Can you work these out from the model? Positions are in its coordinate system, mm. Face numbers are marked on the shaded views. A direction names the side the tool comes from. Give positions to 0.01 mm unless a question says otherwise; leave off trailing zeros. Order: outer loops, then holes, each group sorted by start corner. A loop starts at its lowest first (then second) coordinate and runs counter-clockwise, first axis right, second up. Notation, with made-up numbers: M 67.25,56 L 101.25,56 A28 cw 101.25,74 Z; hole C 72.5,46 d4. An arc over 180 degrees is marked long. Write each question's results on one line, items separated by ' | '.
from build123d import *

# Parameters (mm, degrees)
BOSS_EXTRUDE1_DEPTH     = 25
CUT_EXTRUDE1_DEPTH      = 6
CUT_EXTRUDE1_DEPTH_BACK = 6
SKETCH2_R               = 2.65
SKETCH3_R               = 2.65
CUT_EXTRUDE2_DEPTH      = 91.385151574
CHAMFER1_SIZE           = 10
SKETCH4_R               = 5
CUT_EXTRUDE4_DEPTH      = 6
CHAMFER2_SIZE           = 10
SKETCH5_R               = 5
CUT_EXTRUDE5_DEPTH      = 6


with BuildPart() as part:
    # Sketch1 → Boss-Extrude1 (new body)
    with BuildSketch(Plane(origin=(0, 0, 0), x_dir=(0, 0, -1), z_dir=(1, 0, 0))):
        Polygon((0, 0), (0, 10), (-20, 10), (-20, 14), (0, 14), (0, 84.525), (20, 84.525), (20, 80.525), (4, 80.525), (4, 70), (20, 70), (20, 66), (4, 66), (4, 0), align=None)
    extrude(amount=BOSS_EXTRUDE1_DEPTH)

    # Sketch2 → Cut-Extrude1 (cut, two sides: drawn at the far end of the back side and taken through both)
    with BuildSketch(Plane(origin=(0, 14, 0), x_dir=(1, 0, 0), z_dir=(0, 1, 0)).offset(-CUT_EXTRUDE1_DEPTH_BACK)):
        with Locations(Location((12.5, -10, 0), (0, 0, 90))):
            Circle(SKETCH2_R)
    extrude(amount=CUT_EXTRUDE1_DEPTH + CUT_EXTRUDE1_DEPTH_BACK, mode=Mode.SUBTRACT)

    # Sketch3 → Cut-Extrude2 (cut, through all)
    with BuildSketch(Plane(origin=(0, 84.525, 0), x_dir=(1, 0, 0), z_dir=(0, 1, 0))):
        with Locations(Location((12.5, 14, 0), (0, 0, 270))):
            Circle(SKETCH3_R)
    extrude(amount=-CUT_EXTRUDE2_DEPTH, mode=Mode.SUBTRACT)

    # Chamfer1
    # the kernel refuses this chamfer: 10 mm, written as the material it adds along each edge
    with BuildSketch(Plane(origin=(0, 14, 0), x_dir=(0, -0.027495876610586317, 0.9996219169112968), z_dir=(1, 0, 0))) as chamfer1_piece_1_section:
        Polygon((CHAMFER1_SIZE * 0.999621916911, -CHAMFER1_SIZE * 0.0274958766106), (-CHAMFER1_SIZE * 0.0274958766106, -CHAMFER1_SIZE * 0.999621916911), (0, 0), align=None)
    chamfer1_piece_1 = extrude(amount=25, mode=Mode.PRIVATE)
    chamfer1_piece_1 = chamfer1_piece_1 - Plane(origin=(12.5, 17.333000487, 10), x_dir=(0, 0, -1), z_dir=(0, 1, 0)) * Cylinder(2.65, 90, mode=Mode.PRIVATE)
    add(chamfer1_piece_1)

    # Sketch4 → Cut-Extrude4 (cut)
    with BuildSketch(Plane(origin=(0, 14, 0), x_dir=(1, 0, 0), z_dir=(0, 1, 0))):
        with Locations((12.5, -10)):
            Circle(SKETCH4_R)
    extrude(amount=CUT_EXTRUDE4_DEPTH, mode=Mode.SUBTRACT)

    # Chamfer2
    # the kernel refuses this chamfer: 10 mm, written as the material it adds along each edge
    with BuildSketch(Plane(origin=(0, 66, -4), x_dir=(0, -0.9996219169112968, 0.027495876610586233), z_dir=(1, 0, 0))) as chamfer2_piece_1_section:
        Polygon((CHAMFER2_SIZE * 0.999621916911, CHAMFER2_SIZE * 0.0274958766106), (-CHAMFER2_SIZE * 0.0274958766106, CHAMFER2_SIZE * 0.999621916911), (0, 0), align=None)
    chamfer2_piece_1 = extrude(amount=25, mode=Mode.PRIVATE)
    chamfer2_piece_1 = chamfer2_piece_1 - Plane(origin=(12.5, 62.667000224, -14), x_dir=(0, 0, 1), z_dir=(0, 1, 0)) * Cylinder(2.65, 90, mode=Mode.PRIVATE)
    add(chamfer2_piece_1)

    # Sketch5 → Cut-Extrude5 (cut)
    with BuildSketch(Plane.XZ.offset(-66)):
        with Locations((12.5, -14)):
            Circle(SKETCH5_R)
    extrude(amount=CUT_EXTRUDE5_DEPTH, mode=Mode.SUBTRACT)


solid = part.part
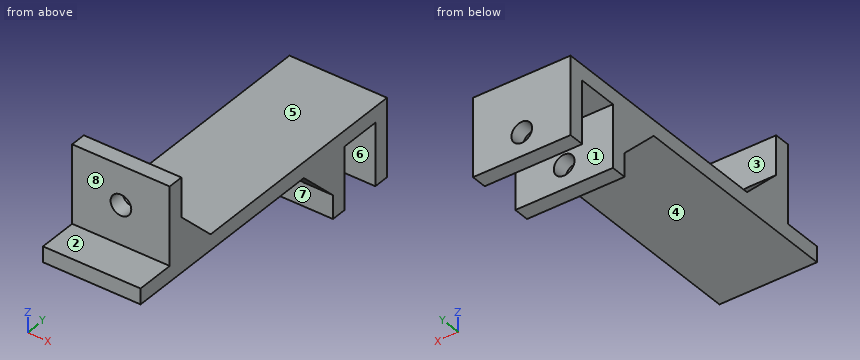
(1) We'd pull the mould along Y, two halves only. Please class the marked faces 1, 2 and 3: +Y half, -Y half, draft (parallel to the pull), parting line (faces both ways), or undercut.
Data:
face 1: undercut | face 2: draft | face 3: +Y half
(2) I need wall thicknesses on L1, parallel to X at y = 68.05, z = -14; L2, parallel to Z at x = 13.75, y = 9; L3, parallel to Y at x = 3.25, z = 5. Which ranges of each line are inside material? Lowest first, please. Write a range as from..to.
Data:
L1: x = 0..9.85, 15.15..25 | L2: z = -4..0 | L3: y = 10..19
(3) Imagine slicing it at B-B, the plane y = 12.5. Write out the boundary of the cut face in (x, z).
Data:
outline: M 0,-4 L 25,-4 L 25,20 L 0,20 Z; hole C 12.5,10 d5.3
(4) Imagine slicing it at A-A, the plane x = 12.5. Count the separate pieces of the cut face and the enclosed holes in it, plus the area to 4 significant figures.
Data:
separate pieces: 4 | enclosed holes: 0 | area: 557.5 mm2
(5) Will these pins go through, and if not, where does the flat tip stop? P1, Ø5, axis at x = 14.5, y = 7, coming from the +Z side; P2, Ø12, axis at x = 8.5, z = 13, coming from the -Y side; P3, Ø1.5, axis at x = 17, z = -15, coming from the -Y side.
Data:
P1: stops at z = 0 | P2: stops at y = 10 | P3: stops at y = 66
(6) Imagine slicing it at D-D, the plane x = 18.5. Write out the boundary of the cut face in (y, z) (3 decimals), plus the area to 3 significant figures.
Data:
outline: M 0,-4 L 56,-4 L 66,-14 L 66,-20 L 70,-20 L 70,-4 L 80.525,-4 L 80.525,-20 L 84.525,-20 L 84.525,0 L 24,0 L 14,10 L 14,20 L 10,20 L 10,0 L 0,0 Z | area: 646 mm2
(7) Imagine slicing it at C-C, the plane z = 9. Write out the boundary of the cut face in (x, y).
Data:
outline: M 0,10 L 10.05,10 L 10.05,14 L 7.6,14 L 7.6,15 L 0,15 Z; M 14.95,10 L 25,10 L 25,15 L 17.4,15 L 17.4,14 L 14.95,14 Z
(8) For the marked faces 4, 5, 6, 7 and 8, which set-ups out of +Z, -Z, +X, -X, +Y, -Y let a thin tool reach every point of the face, with its end or its side?
Data:
face 4: -Z, +X, -X, -Y | face 5: +Z, +X, -X, +Y | face 6: -Z, +X, -X | face 7: -Z, -Y | face 8: +Z, +X, -X, -Y
